Design review of the part built by this model. Coordinates are the model's own, in mm. Give positions to 0.01 mm unless a question says otherwise; leave off trailing zeros. Write each loop counter-clockwise with the first axis right and the second up, starting at its lowest first coordinate (ties: lowest second). Pieces come first, ordered by that corner, then holes. Notation, with made-up numbers: (-11.5, 9.25) - (26.5, 9.25) arc R15 ccw to (26.5, 31.25) - close; hole circle Ø5 at (48.5, -12). An arc over 180 degrees is marked (long way). Use a Markdown table: item, result. Add a question column.
```python
from build123d import *

# Parameters (mm, degrees)
SKETCH1_R           = 4.75
SKETCH1_R_2         = 4.25
BOSS_EXTRUDE1_DEPTH = 1
SKETCH2_R           = 4.5
CUT_EXTRUDE1_DEPTH  = 0.5
FILLET1_R           = 1
FILLET2_R           = 0.1


with BuildPart() as part:
    # Sketch1 → Boss-Extrude1 (new body)
    with BuildSketch(Plane(origin=(0, 0, 0), x_dir=(1, 0, 0), z_dir=(0, 1, 0))):
        with Locations(Location((0, 0, 0), (0, 0, 270))):
            Circle(SKETCH1_R)
        with Locations(Location((0, 0, 0), (0, 0, 270))):
            Circle(SKETCH1_R_2, mode=Mode.SUBTRACT)
    extrude(amount=BOSS_EXTRUDE1_DEPTH)

    # Sketch2 → Cut-Extrude1 (cut)
    with BuildSketch(Plane(origin=(0, 1, 0), x_dir=(1, 0, 0), z_dir=(0, 1, 0))):
        with Locations(Location((0, 0, 0), (0, 0, 270))):
            Circle(SKETCH2_R)
    extrude(amount=-CUT_EXTRUDE1_DEPTH, mode=Mode.SUBTRACT)

    # Fillet1
    # the kernel refuses this fillet: 1 mm, written as the material it takes off along each edge
    with BuildSketch(Plane(origin=(0, 0, 0), x_dir=(0, 0, 1), z_dir=(-1, 0, 0))) as fillet1_piece_1:
        with BuildLine():
            CenterArc((3.75, 0.866025404), FILLET1_R, 300, 60)
            Line((4.25, 0), (4.26, -0.017320508))
            ThreePointArc((4.26, -0.017320508), (4.5, -0.02), (4.75, -0.02))
            Line((4.75, -0.02), (4.77, 0))
            Line((4.77, 0), (4.77, 0.866025404))
            Line((4.77, 0.866025404), (4.75, 0.866025404))
        make_face()
    revolve(axis=Axis((0, 0, 0), (0, 1, 0)), mode=Mode.SUBTRACT)

    # Fillet2
    fillet2_edges = [part.edges().sort_by_distance(p)[0] for p in [
        (0, 1, -4.75),
    ]]
    fillet(fillet2_edges, radius=FILLET2_R)


solid = part.part
```
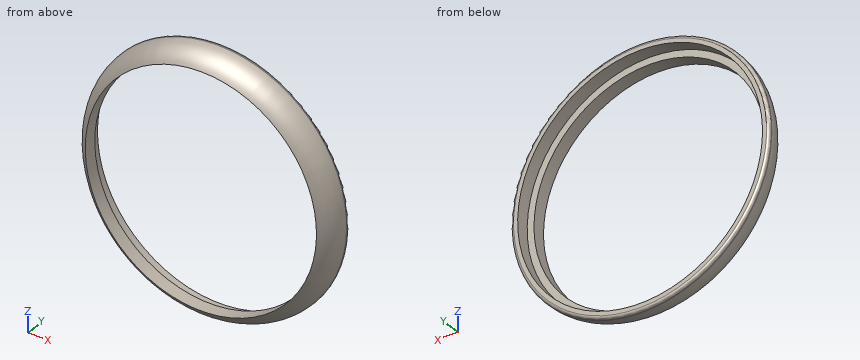
(1) For line 1 along X through (y, z) = (0.35, 0); line 2 along X through (y, z) = (0.6, 3.5); line 3 along Z through (x, y) = (-1.5, 0.3), list the stretches that pass through material, from the lowest coordinate up.
(2) Insertion check: pin 1 (5 mm diameter, centred on x = 0, z = 0, fed in from -Y). The pin has a flat end and moves straight along its axis. Give the tip position at first contact, or say it passes through.
(3) Add section C-C (y = 0.65). State the section outline as (x, z) points.
Answers follow:
| question | item | result |
|---|---|---|
| 1 | line 1 | -4.61 to -4.25, 4.25 to 4.61 |
| 1 | line 2 | -3.16 to -2.83, 2.83 to 3.16 |
| 1 | line 3 | -4.32 to -3.98, 3.98 to 4.32 |
| 2 | pin 1 | through |
| 3 | outline | circle Ø9.45 at (0, 0); hole circle Ø9 at (0, 0) |
